Read the model definition and answer for the solid it produces. Units are mm, in the model's axes. Coordinates: 2 decimals unless noted, no trailing zeros. Write each loop counter-clockwise with the first axis right and the second up, starting at its lowest first coordinate (ties: lowest second). Pieces come first, ordered by that corner, then holes. Notation, with made-up numbers: (-28, -21.75) -> (-15, -21.75) arc R18 ccw to (-15, 4.25) -> close; hole circle Ø7 at (30, -32). An arc over 180 degrees is marked (long way). Answer as a JSON object with one key per item and string values. Group by question number.
(1) Find section C-C (y = 56). Give the vertices of the cut face in (x, z), then the cut area to 3 significant figures.
(2) Find section D-D (y = 64.5). Give the vertices of the cut face in (x, z), then the cut area to 3 significant figures.
(3) Find section B-B (x = 0). Give the vertices of the cut face in (y, z), then the cut area to 3 significant figures.
(4) Straight lines are drawn through the part: L1, parallel to X at y = 60, z = 1.8; L2, parallel to Y at x = -39, z = 1.25; L3, parallel to Y at x = 25, z = 0.7. For each, find the intervals that lie inside material, in ascending order.
(5) Find section A-A (y = -1.5). Give the vertices of the cut face in (x, z), then the cut area to 3 significant figures.
(6) Flat-ended cylindrical pins translate along their axes: P1, Ø3.5, axis at x = 39.82, y = 49.5, coming from the +Z side; P2, Ø0.9, axis at x = 39, z = 1, coming from the -Y side. Find the tip coordinate at first contact, or state that the pin passes through.
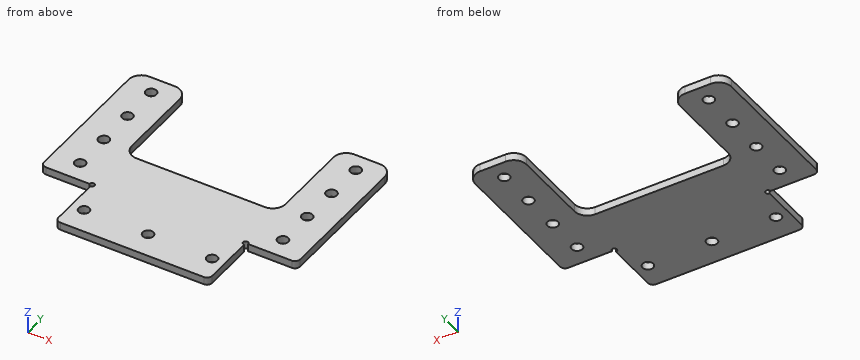
from build123d import *

# Parameters (mm, degrees)
SKETCH1_W           = 60
SKETCH1_H           = 23
BOSS_EXTRUDE1_DEPTH = 3
BOSS_EXTRUDE2_DEPTH = 3
SKETCH3_R           = 1
CUT_EXTRUDE1_DEPTH  = 88.299770905
FILLET1_R           = 2
SKETCH4_R           = 2.1
CUT_EXTRUDE2_DEPTH  = 88.299770905
SKETCH5_R           = 2.1
CUT_EXTRUDE3_DEPTH  = 88.299770905
FILLET2_R           = 5


with BuildPart() as part:
    # Sketch1 → Boss-Extrude1 (new body)
    with BuildSketch(Plane.XY):
        Rectangle(SKETCH1_W, SKETCH1_H)
    extrude(amount=BOSS_EXTRUDE1_DEPTH)

    # Sketch2 → Boss-Extrude2 (add)
    with BuildSketch(Plane.XY.offset(3)):
        Polygon((50, 11.5), (-50, 11.5), (-50, 71.5), (-30, 71.5), (-30, 31.5), (30, 31.5), (30, 71.5), (50, 71.5), align=None)
    extrude(amount=-BOSS_EXTRUDE2_DEPTH)

    # Sketch3 → Cut-Extrude1 (cut, through all)
    with BuildSketch(Plane.XY.offset(3)):
        with Locations((-30, 11.5)):
            Circle(SKETCH3_R)
        with Locations((30, 11.5)):
            Circle(SKETCH3_R)
    extrude(amount=-CUT_EXTRUDE1_DEPTH, mode=Mode.SUBTRACT)

    # Fillet1
    fillet1_edges = [part.edges().sort_by_distance(p)[0] for p in [
        (50, 11.5, 1.5),
        (-50, 11.5, 1.5),
        (30, -11.5, 1.5),
        (-30, -11.5, 1.5),
    ]]
    fillet(fillet1_edges, radius=FILLET1_R)

    # Sketch4 → Cut-Extrude2 (cut, through all)
    with BuildSketch(Plane.XY.offset(3)):
        with Locations((-25, -1.5)):
            Circle(SKETCH4_R)
        with Locations((0, -1.5)):
            Circle(SKETCH4_R)
        with Locations((25, -1.5)):
            Circle(SKETCH4_R)
    extrude(amount=-CUT_EXTRUDE2_DEPTH, mode=Mode.SUBTRACT)

    # Sketch5 → Cut-Extrude3 (cut, through all)
    with BuildSketch(Plane.XY.offset(3)):
        with Locations((-39.941666667, 64.5)):
            Circle(SKETCH5_R)
        with Locations((-39.816671007, 49.500520806)):
            Circle(SKETCH5_R)
        with Locations((-39.691675347, 34.501041612)):
            Circle(SKETCH5_R)
        with Locations((-39.566679687, 19.501562419)):
            Circle(SKETCH5_R)
        with Locations(Location((39.566679687, 19.501562419, 0), (0, 0, 180))):
            Circle(SKETCH5_R)
        with Locations(Location((39.691675347, 34.501041612, 0), (0, 0, 180))):
            Circle(SKETCH5_R)
        with Locations(Location((39.816671007, 49.500520806, 0), (0, 0, 180))):
            Circle(SKETCH5_R)
        with Locations(Location((39.941666667, 64.5, 0), (0, 0, 180))):
            Circle(SKETCH5_R)
    extrude(amount=-CUT_EXTRUDE3_DEPTH, mode=Mode.SUBTRACT)

    # Fillet2
    fillet2_edges = [part.edges().sort_by_distance(p)[0] for p in [
        (50, 71.5, 1.5),
        (30, 71.5, 1.5),
        (30, 31.5, 1.5),
        (-30, 31.5, 1.5),
        (-30, 71.5, 1.5),
        (-50, 71.5, 1.5),
    ]]
    fillet(fillet2_edges, radius=FILLET2_R)


solid = part.part
Results below:
{
 "1": {"outline": "(-50, 0) -> (-30, 0) -> (-30, 3) -> (-50, 3) -> close; (30, 0) -> (50, 0) -> (50, 3) -> (30, 3) -> close", "area": "120 mm2"},
 "2": {"outline": "(-50, 0) -> (-42.04, 0) -> (-42.04, 3) -> (-50, 3) -> close; (-37.84, 0) -> (-30, 0) -> (-30, 3) -> (-37.84, 3) -> close; (30, 0) -> (37.84, 0) -> (37.84, 3) -> (30, 3) -> close; (42.04, 0) -> (50, 0) -> (50, 3) -> (42.04, 3) -> close", "area": "94.8 mm2"},
 "3": {"outline": "(-11.5, 0) -> (-3.6, 0) -> (-3.6, 3) -> (-11.5, 3) -> close; (0.6, 0) -> (31.5, 0) -> (31.5, 3) -> (0.6, 3) -> close", "area": "116 mm2"},
 "4": {"L1": "x = -50 to -30, 30 to 50", "L2": "y = 11.5 to 17.48, 21.52 to 32.52, 36.48 to 47.57, 51.44 to 62.62, 66.38 to 71.5", "L3": "y = -11.5 to -3.6, 0.6 to 31.5"},
 "5": {"outline": "(-30, 0) -> (-27.1, 0) -> (-27.1, 3) -> (-30, 3) -> close; (-22.9, 0) -> (-2.1, 0) -> (-2.1, 3) -> (-22.9, 3) -> close; (2.1, 0) -> (22.9, 0) -> (22.9, 3) -> (2.1, 3) -> close; (27.1, 0) -> (30, 0) -> (30, 3) -> (27.1, 3) -> close", "area": "142 mm2"},
 "6": {"P1": "passes through", "P2": "stops at y = 11.5"}
}
